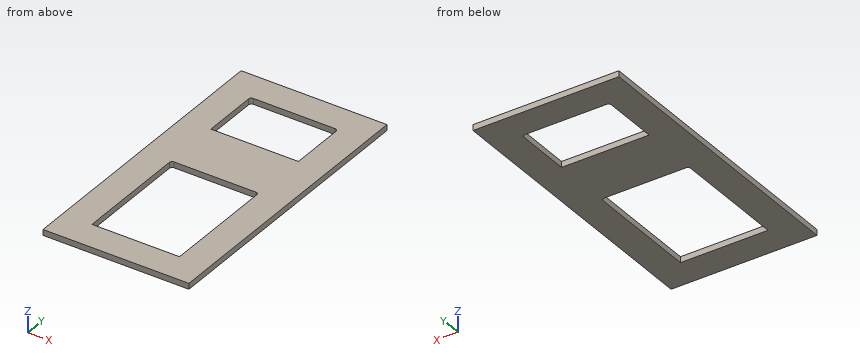
```python
from build123d import *

# Parameters (mm, degrees)
BOX001_W     = 30
BOX001_H     = 40
BOX001_DEPTH = 10
BOX002_W     = 30
BOX002_H     = 20
BOX002_DEPTH = 10
BOX_W        = 50
BOX_H        = 100
BOX_DEPTH    = 2
FILLET001_R  = 1
FILLET002_R  = 1


with BuildPart() as cubo001:
    # Box001 → Box001 (new body)
    with BuildSketch(Plane(origin=(10, 10, 0), x_dir=(1, 0, 0), z_dir=(0, 0, 1))):
        with Locations((15, 20)):
            Rectangle(BOX001_W, BOX001_H)
    extrude(amount=BOX001_DEPTH)


with BuildPart() as fusion:
    # Box002 → Box002 (new body)
    with BuildSketch(Plane(origin=(10, 70, 0), x_dir=(1, 0, 0), z_dir=(0, 0, 1))):
        with Locations((15, 10)):
            Rectangle(BOX002_W, BOX002_H)
    extrude(amount=BOX002_DEPTH)

    # Fusion: union Cubo001
    add(cubo001.part)


with BuildPart() as fillet002:
    # Box → Box (new body)
    with BuildSketch(Plane.XY):
        with Locations((25, 50)):
            Rectangle(BOX_W, BOX_H)
    extrude(amount=BOX_DEPTH)

    # Cut: cut Fusion
    add(fusion.part, mode=Mode.SUBTRACT)

    # Fillet001
    fillet001_edges = [fillet002.edges().sort_by_distance(p)[0] for p in [
        (10, 50, 1),
        (10, 90, 1),
    ]]
    fillet(fillet001_edges, radius=FILLET001_R)

    # Fillet002
    fillet002_edges = [fillet002.edges().sort_by_distance(p)[0] for p in [
        (40, 50, 1),
        (40, 90, 1),
    ]]
    fillet(fillet002_edges, radius=FILLET002_R)


solid = fillet002.part
```
Geometry: final body of the model. Coordinates: model frame, mm. Coordinates: 2 decimals unless noted, no trailing zeros. Loops run counter-clockwise (first coordinate to the right, second up) from the corner with the lowest first, then second, coordinate; pieces in that order, holes last. Notation, with made-up numbers: (88.5, 60.5) -> (103.5, 60.5) arc R13 ccw to (103.5, 84.5) -> close; hole circle Ø11 at (28.25, 83). An arc over 180 degrees is marked (long way). Use a Markdown table: item, result. Add a question column.
(1) Section query A-A, the plane x = 17. Return loops of the section in (y, z), plus the area to 3 significant figures.
(2) Section query B-B, the plane z = 0.35. Return loops of the section in (x, y), plus the area to 3 significant figures.
(3) Line query: line 1 along Y through (x, z) = (25.5, 1.05); line 2 along X through (y, z) = (89, 0.75). Output: solid intervals per line, ascending.
(4) Section query C-C, the plane y = 31.5. Return loops of the section in (x, z), plus the area to 3 significant figures.
Answer:
| question | item | result |
|---|---|---|
| 1 | outline | (0, 0) -> (10, 0) -> (10, 2) -> (0, 2) -> close; (50, 0) -> (70, 0) -> (70, 2) -> (50, 2) -> close; (90, 0) -> (100, 0) -> (100, 2) -> (90, 2) -> close |
| 1 | area | 80.0 mm^2 |
| 2 | outline | (0, 0) -> (50, 0) -> (50, 100) -> (0, 100) -> close; hole (10, 10) -> (40, 10) -> (40, 49) arc R1 ccw to (39, 50) -> (11, 50) arc R1 ccw to (10, 49) -> close; hole (10, 70) -> (40, 70) -> (40, 89) arc R1 ccw to (39, 90) -> (11, 90) arc R1 ccw to (10, 89) -> close |
| 2 | area | 3,200 mm^2 |
| 3 | line 1 | y = 0 to 10, 50 to 70, 90 to 100 |
| 3 | line 2 | x = 0 to 10, 40 to 50 |
| 4 | outline | (0, 0) -> (10, 0) -> (10, 2) -> (0, 2) -> close; (40, 0) -> (50, 0) -> (50, 2) -> (40, 2) -> close |
| 4 | area | 40.0 mm^2 |
